```python
from build123d import *

# Parameters (mm, degrees)
CYLINDER004_R        = 1.5
CYLINDER004_DEPTH    = 10
CYLINDER003_R        = 1.5
CYLINDER003_DEPTH    = 10
CYLINDER002_R        = 1.5
CYLINDER002_DEPTH    = 10
CYLINDER001_R        = 1.5
CYLINDER001_DEPTH    = 10
BOX007_W             = 40
BOX007_H             = 1
BOX007_DEPTH         = 10.5
BOX006_W             = 40
BOX006_H             = 1
BOX006_DEPTH         = 10.5
BOX005_W             = 3
BOX005_H             = 25
BOX005_DEPTH         = 10
BOX004_W             = 2
BOX004_H             = 16
BOX004_DEPTH         = 9
BOX003_W             = 2
BOX003_H             = 13
BOX003_DEPTH         = 5
BOX002_W             = 2
BOX002_H             = 25
BOX002_DEPTH         = 9
BOX001_W             = 69
BOX001_H             = 25
BOX001_DEPTH         = 13
CYLINDER_R           = 3
CYLINDER_DEPTH       = 2
CYLINDER_PITCH_ANGLE = 90
BOX_W                = 80
BOX_H                = 35
BOX_DEPTH            = 8.5


with BuildPart() as cylinder004:
    # Cylinder004 → Cylinder004 (new body)
    with BuildSketch(Plane(origin=(2.5, 32.5, 0), x_dir=(1, 0, 0), z_dir=(0, 0, 1))):
        Circle(CYLINDER004_R)
    extrude(amount=CYLINDER004_DEPTH)


with BuildPart() as cylinder003:
    # Cylinder003 → Cylinder003 (new body)
    with BuildSketch(Plane(origin=(77.5, 32.5, 0), x_dir=(1, 0, 0), z_dir=(0, 0, 1))):
        Circle(CYLINDER003_R)
    extrude(amount=CYLINDER003_DEPTH)


with BuildPart() as cylinder002:
    # Cylinder002 → Cylinder002 (new body)
    with BuildSketch(Plane(origin=(77.5, 2.5, 0), x_dir=(1, 0, 0), z_dir=(0, 0, 1))):
        Circle(CYLINDER002_R)
    extrude(amount=CYLINDER002_DEPTH)


with BuildPart() as cylinder001:
    # Cylinder001 → Cylinder001 (new body)
    with BuildSketch(Plane(origin=(2.5, 2.5, 0), x_dir=(1, 0, 0), z_dir=(0, 0, 1))):
        Circle(CYLINDER001_R)
    extrude(amount=CYLINDER001_DEPTH)


with BuildPart() as box007:
    # Box007 → Box007 (new body)
    with BuildSketch(Plane(origin=(20, 1, 0), x_dir=(1, 0, 0), z_dir=(0, 0, 1))):
        with Locations((20, 0.5)):
            Rectangle(BOX007_W, BOX007_H)
    extrude(amount=BOX007_DEPTH)


with BuildPart() as box006:
    # Box006 → Box006 (new body)
    with BuildSketch(Plane(origin=(20, 33, 0), x_dir=(1, 0, 0), z_dir=(0, 0, 1))):
        with Locations((20, 0.5)):
            Rectangle(BOX006_W, BOX006_H)
    extrude(amount=BOX006_DEPTH)


with BuildPart() as box005:
    # Box005 → Box005 (new body)
    with BuildSketch(Plane(origin=(2, 5, 2), x_dir=(1, 0, 0), z_dir=(0, 0, 1))):
        with Locations((1.5, 12.5)):
            Rectangle(BOX005_W, BOX005_H)
    extrude(amount=BOX005_DEPTH)


with BuildPart() as box004:
    # Box004 → Box004 (new body)
    with BuildSketch(Plane(origin=(74, 9.5, 4), x_dir=(1, 0, 0), z_dir=(0, 0, 1))):
        with Locations((1, 8)):
            Rectangle(BOX004_W, BOX004_H)
    extrude(amount=BOX004_DEPTH)


with BuildPart() as u:
    # Box003 → Box003 (new body)
    with BuildSketch(Plane(origin=(78, 11, 6), x_dir=(1, 0, 0), z_dir=(0, 0, 1))):
        with Locations((1, 6.5)):
            Rectangle(BOX003_W, BOX003_H)
    extrude(amount=BOX003_DEPTH)


with BuildPart() as box002:
    # Box002 → Box002 (new body)
    with BuildSketch(Plane(origin=(76, 5, 4), x_dir=(1, 0, 0), z_dir=(0, 0, 1))):
        with Locations((1, 12.5)):
            Rectangle(BOX002_W, BOX002_H)
    extrude(amount=BOX002_DEPTH)


with BuildPart() as box001:
    # Box001 → Box001 (new body)
    with BuildSketch(Plane(origin=(5, 5, 2), x_dir=(1, 0, 0), z_dir=(0, 0, 1))):
        with Locations((34.5, 12.5)):
            Rectangle(BOX001_W, BOX001_H)
    extrude(amount=BOX001_DEPTH)


with BuildPart() as cylinder:
    # Cylinder → Cylinder (new body)
    with BuildSketch(Plane.XY):
        Circle(CYLINDER_R)
    extrude(amount=CYLINDER_DEPTH)


with BuildPart() as cylinder_1:
    # Cylinder pitch: moved
    add(cylinder.part.rotate(Axis((0, 0, 0), (0, 1, 0)), CYLINDER_PITCH_ANGLE))


with BuildPart() as cylinder_2:
    # Cylinder placement: moved
    add(cylinder_1.part.moved(Location((0, 17.5, 8.5))))


with BuildPart() as cut009:
    # Box → Box (new body)
    with BuildSketch(Plane.XY):
        with Locations((40, 17.5)):
            Rectangle(BOX_W, BOX_H)
    extrude(amount=BOX_DEPTH)

    # Cut: cut Cylinder
    add(cylinder_2.part, mode=Mode.SUBTRACT)

    # Cut001: cut Box001
    add(box001.part, mode=Mode.SUBTRACT)

    # Cut002: cut Box002
    add(box002.part, mode=Mode.SUBTRACT)

    add(u.part, mode=Mode.SUBTRACT)

    # Cut004: cut Box004
    add(box004.part, mode=Mode.SUBTRACT)

    # Cut005: cut Box005
    add(box005.part, mode=Mode.SUBTRACT)

    # Fusion: union Box006
    add(box006.part)

    # Fusion001: union Box007
    add(box007.part)

    # Cut006: cut Cylinder001
    add(cylinder001.part, mode=Mode.SUBTRACT)

    # Cut007: cut Cylinder002
    add(cylinder002.part, mode=Mode.SUBTRACT)

    # Cut008: cut Cylinder003
    add(cylinder003.part, mode=Mode.SUBTRACT)

    # Cut009: cut Cylinder004
    add(cylinder004.part, mode=Mode.SUBTRACT)


solid = cut009.part
```
Input: part model. Units: mm. Frame: model coordinates. A direction names the side the tool comes from. Round coordinates to 2 decimals unless told otherwise and drop trailing zeros. Order: outer loops, then holes, each group sorted by start corner. A loop starts at its lowest first (then second) coordinate and runs counter-clockwise, first axis right, second up. Notation, with made-up numbers: (-18, 13.5) - (20, 13.5) arc R15 ccw to (20, 32.5) - close; hole circle Ø10 at (87.25, -20.5). An arc over 180 degrees is marked (long way). One line per question, with ' | ' between items. Start each with the question number.
1) Contact query for flat-ended pins moving along their axis: P1, Ø2, axis at x = 79, z = 7.5, coming from the -Y side; P2, Ø12, axis at x = 42, y = 21, coming from the +Z side; P3, Ø1.1, axis at y = 1.5, z = 9.5, coming from the -X side; P4, Ø11.5, axis at x = 31.5, y = 27, coming from the +Z side. Output: stop coordinate, or through.
2) Cut plane A-A, the plane y = 17.5. Return the cut outline in (x, z).
3) Ray query, probe 1 along X at (y, z) = (2.5, 2.75); probe 2 along Y at (x, z) = (77.5, 5.25); probe 3 along X at (y, z) = (29, 8.25). Return the intervals inside material, ascending.
4) Set-up query: faces 1 (the flat face through (79, 11, 7)), 2 (the flat face through (78, 17.3, 5.7)), 3 (the flat face through (40, 1, 9)). Return all of +Z, -Z, +X, -X, +Y, -Y with unobstructed straight access to the full face (end or side cutting, diameter ignored); none if empty.
5) Pull-direction query (Y, two-part tool) for faces 4 (the flat face through (39, 35, 4)), 5 (the flat face through (0, 17, 4)), 6 (the flat face through (76, 7, 6)), 7 (the flat face through (77, 5, 6)); classes: +Y half, -Y half, draft (parallel to the pull), parting line (faces both ways), or undercut.
6) Cut plane B-B, the plane x = 7. Return the cut outline in (y, z).
7) Cut plane D-D, the plane x = 42.5. Return the cut outline in (y, z), then the cut area to 3 significant figures.
8) Cut plane C-C, the plane y = 27. Return the cut outline in (x, z), then the cut area to 3 significant figures.
Worked out:
1) P1: stops at y = 0 | P2: stops at z = 2 | P3: stops at x = 20 | P4: stops at z = 8.5
2) outline: (0, 0) - (80, 0) - (80, 6) - (78, 6) - (78, 4) - (74, 4) - (74, 2) - (2, 2) - (2, 5.5) - (0, 5.5) - close
3) probe 1: x = 0 to 1, 4 to 76, 79 to 80 | probe 2: y = 0 to 1, 4 to 5, 30 to 31, 34 to 35 | probe 3: x = 0 to 2, 74 to 76, 78 to 80
4) face 1: +Z, +X | face 2: +Z | face 3: +Z, +X, -X, -Y
5) face 4: +Y half | face 5: draft | face 6: undercut | face 7: undercut
6) outline: (0, 0) - (35, 0) - (35, 8.5) - (30, 8.5) - (30, 2) - (5, 2) - (5, 8.5) - (0, 8.5) - close
7) outline: (0, 0) - (35, 0) - (35, 8.5) - (34, 8.5) - (34, 10.5) - (33, 10.5) - (33, 8.5) - (30, 8.5) - (30, 2) - (5, 2) - (5, 8.5) - (2, 8.5) - (2, 10.5) - (1, 10.5) - (1, 8.5) - (0, 8.5) - close | area: 139 mm^2
8) outline: (0, 0) - (80, 0) - (80, 8.5) - (78, 8.5) - (78, 4) - (76, 4) - (76, 8.5) - (74, 8.5) - (74, 2) - (2, 2) - (2, 8.5) - (0, 8.5) - close | area: 203 mm^2
